Work out the finished part from the listing and answer in its coordinate system (mm). Face numbers are marked on the shaded views. Coordinates: 2 decimals unless noted, no trailing zeros. Loops run counter-clockwise (first coordinate to the right, second up) from the corner with the lowest first, then second, coordinate; pieces in that order, holes last. Notation, with made-up numbers: (61.5, 72) -> (110.5, 72) arc R24 ccw to (110.5, 89) -> close; hole circle Ø7 at (53.5, -26.5). An arc over 180 degrees is marked (long way). Use a Markdown table: item, result.
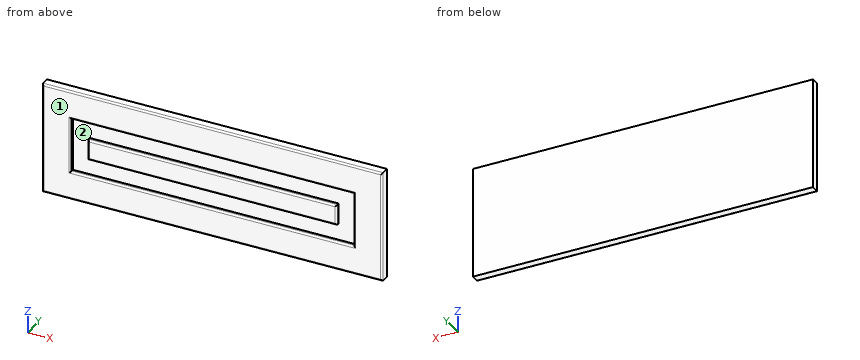
from build123d import *

# Parameters (mm, degrees)
F0_W      = 44.656470418
F0_H      = 33.8078811765
F1_DEPTH  = 16
F2_DEPTH  = 796
F3_DEPTH  = 196
F4_W      = 68.9578056335
F4_H      = 493.6993122101
F5_DEPTH  = 7
F6_DEPTH  = 9.7
F7_DEPTH  = 99.33
F8_DEPTH  = 99.33
F9_DEPTH  = 17.34
F10_DEPTH = 102.97
F11_W     = 35.2807044983
F11_H     = 492.0964837074
F12_DEPTH = 7
F13_DEPTH = 37.27
F14_DEPTH = 6.58
F15_DEPTH = 106.63
F16_DEPTH = 5.87
F17_DEPTH = 200
F18_DEPTH = 200
F19_DEPTH = 200
F20_DEPTH = 200
F21_DEPTH = 200
F22_DEPTH = 200
F23_DEPTH = 600
F24_DEPTH = 600
F25_DEPTH = 600
F26_R     = 3


with BuildPart() as f1:
    # F0 (on Front) → F1 (new body)
    with BuildSketch(Plane.XZ):
        with Locations((22.328235209, 16.9039405882)):
            Rectangle(F0_W, F0_H)
    extrude(amount=F1_DEPTH)

    # F2 (add): a face of the model
    f2_faces = [f1.faces().sort_by_distance(p)[0] for p in [
        (22.328235209, -8, 0),
    ]]
    extrude(f2_faces, amount=-F2_DEPTH)

    # F3 (add): a face of the model
    f3_faces = [f1.faces().sort_by_distance(p)[0] for p in [
        (0, -8, 398),
    ]]
    extrude(f3_faces, amount=-F3_DEPTH)

    # F4 (on face) → F5 (cut)
    with BuildSketch(Plane.XZ.offset(16)):
        with Locations((94.1769480705, 399.8196721077)):
            Rectangle(F4_W, F4_H)
    extrude(amount=-F5_DEPTH, mode=Mode.SUBTRACT)

    # F6 (cut): a face of the model
    f6_faces = [f1.faces().sort_by_distance(p)[0] for p in [
        (59.6980452538, -12.5, 399.8196721077),
    ]]
    extrude(f6_faces, amount=-F6_DEPTH, mode=Mode.SUBTRACT)

    # F7 (add): a face of the model
    f7_faces = [f1.faces().sort_by_distance(p)[0] for p in [
        (89.3269480705, -12.5, 646.6693282127),
    ]]
    extrude(f7_faces, amount=-F7_DEPTH)

    # F8 (cut): a face of the model
    f8_faces = [f1.faces().sort_by_distance(p)[0] for p in [
        (89.3269480705, -12.5, 646.6693282127),
    ]]
    extrude(f8_faces, amount=-F8_DEPTH, mode=Mode.SUBTRACT)

    # F9 (cut): a face of the model
    f9_faces = [f1.faces().sort_by_distance(p)[0] for p in [
        (128.6558508873, -12.5, 449.4846721077),
    ]]
    extrude(f9_faces, amount=-F9_DEPTH, mode=Mode.SUBTRACT)

    # F10 (cut): a face of the model
    f10_faces = [f1.faces().sort_by_distance(p)[0] for p in [
        (97.9969480705, -12.5, 152.9700160027),
    ]]
    extrude(f10_faces, amount=-F10_DEPTH, mode=Mode.SUBTRACT)

    # F11 (on face) → F12 (join)
    with BuildSketch(Plane.XZ.offset(9)):
        with Locations((91.7714834213, 432.6795041561)):
            Rectangle(F11_W, F11_H)
    extrude(amount=F12_DEPTH)

    # F13 (add): a face of the model
    f13_faces = [f1.faces().sort_by_distance(p)[0] for p in [
        (91.7714834213, -12.5, 678.7277460098),
    ]]
    extrude(f13_faces, amount=F13_DEPTH)

    # F14 (add): a face of the model
    f14_faces = [f1.faces().sort_by_distance(p)[0] for p in [
        (109.4118356705, -12.5, 451.3145041561),
    ]]
    extrude(f14_faces, amount=F14_DEPTH)

    # F15 (add): a face of the model
    f15_faces = [f1.faces().sort_by_distance(p)[0] for p in [
        (95.0614834213, -12.5, 186.6312623024),
    ]]
    extrude(f15_faces, amount=F15_DEPTH)

    # F16 (cut): a face of the model
    f16_faces = [f1.faces().sort_by_distance(p)[0] for p in [
        (74.1311311722, -12.5, 397.9995041561),
    ]]
    extrude(f16_faces, amount=-F16_DEPTH, mode=Mode.SUBTRACT)

    # F17 (add): a face of the model
    f17_faces = [f1.faces().sort_by_distance(p)[0] for p in [
        (196, -8, 398),
    ]]
    extrude(f17_faces, amount=F17_DEPTH)

    # F18 (cut): a face of the model
    f18_faces = [f1.faces().sort_by_distance(p)[0] for p in [
        (145.9958508873, -12.5, 397.9996721077),
    ]]
    extrude(f18_faces, amount=-F18_DEPTH, mode=Mode.SUBTRACT)

    # F19 (add): a face of the model
    f19_faces = [f1.faces().sort_by_distance(p)[0] for p in [
        (115.9918356705, -12.5, 397.9995041561),
    ]]
    extrude(f19_faces, amount=F19_DEPTH)

    # F20 (add): a face of the model
    f20_faces = [f1.faces().sort_by_distance(p)[0] for p in [
        (396, -8, 398),
    ]]
    extrude(f20_faces, amount=F20_DEPTH)

    # F21 (cut): a face of the model
    f21_faces = [f1.faces().sort_by_distance(p)[0] for p in [
        (345.9958508873, -12.5, 397.9996721077),
    ]]
    extrude(f21_faces, amount=-F21_DEPTH, mode=Mode.SUBTRACT)

    # F22 (add): a face of the model
    f22_faces = [f1.faces().sort_by_distance(p)[0] for p in [
        (315.9918356705, -12.5, 397.9995041561),
    ]]
    extrude(f22_faces, amount=F22_DEPTH)

    # F23 (cut): a face of the model
    f23_faces = [f1.faces().sort_by_distance(p)[0] for p in [
        (297.9964834213, -12.5, 80.0012623024),
    ]]
    extrude(f23_faces, amount=-F23_DEPTH, mode=Mode.SUBTRACT)

    # F24 (add): a face of the model
    f24_faces = [f1.faces().sort_by_distance(p)[0] for p in [
        (297.9969480705, -12.5, 50.0000160027),
    ]]
    extrude(f24_faces, amount=F24_DEPTH)

    # F25 (cut): a face of the model
    f25_faces = [f1.faces().sort_by_distance(p)[0] for p in [
        (298, -8, 0),
    ]]
    extrude(f25_faces, amount=-F25_DEPTH, mode=Mode.SUBTRACT)

    # F26
    f26_edges = [f1.edges().sort_by_distance(p)[0] for p in [
        (0, -16, 698),
        (298, -16, 796),
        (596, -16, 698),
        (298, -16, 600),
        (49.998045, -16, 697.999672),
        (297.996948, -16, 650.000016),
        (297.996948, -16, 745.999328),
        (545.995851, -16, 697.999672),
        (297.996483, -16, 715.997746),
        (515.991836, -16, 697.999504),
        (297.996483, -16, 680.001262),
        (80.001131, -16, 697.999504),
    ]]
    fillet(f26_edges, radius=F26_R)


solid = f1.part
Q1. Section A-A on x = 356 is taken. Determine the outline of the cut face in (y, z), and give its area (3 significant figures).
Solved:
| item | result |
|---|---|
| outline | (-16, 603) arc R3 ccw to (-13, 600) -> (0, 600) -> (0, 796) -> (-13, 796) arc R3 ccw to (-16, 793) -> (-16, 749) arc R3 ccw to (-13, 746) -> (-9, 746) -> (-9, 716) -> (-13, 716) arc R3 ccw to (-16, 713) -> (-16, 683) arc R3 ccw to (-13, 680) -> (-9, 680) -> (-9, 650) -> (-13, 650) arc R3 ccw to (-16, 647) -> close |
| area | 2,700 mm² |
Q2. Consider line 1 (Z direction, x = 302, y = -10); line 2 (Z direction, x = 517, y = -12); line 3 (X direction, y = -11, z = 701). Determine where each line is inside the solid, lowest interval first. Write a range as [from, to].
Solved:
| item | result |
|---|---|
| line 1 | [600, 650], [680, 716], [746, 796] |
| line 2 | [600, 650], [746, 796] |
| line 3 | [0, 50], [80, 515.99], [546, 596] |
Q3. Determine the mould class of the marked faces 1 and 2 for opening direction Z: pulls with the +Z half, pulls with the -Z half, needs draft (parallel to the pull), parting line crosses it, or undercut.
Solved:
| item | result |
|---|---|
| face 1 | needs draft |
| face 2 | undercut |
Q4. Given pin 1 Ø10 at (x, z) = (97.5, 665.5) entering from -Y; pin 2 Ø10 at (x, z) = (511, 674.5) entering from +Y, each flat-ended and moving along its own axis, determine where each tip first touches the part or whether it passes through.
Solved:
| item | result |
|---|---|
| pin 1 | y = -9 |
| pin 2 | y = 0 |
